Input: part model. Units: mm. Frame: model coordinates. Face numbers are marked on the shaded views. A direction names the side the tool comes from. Give positions to 0.01 mm unless a question says otherwise; leave off trailing zeros. Loops run counter-clockwise (first coordinate to the right, second up) from the corner with the lowest first, then second, coordinate; pieces in that order, holes last. Notation, with made-up numbers: (-30.5, 2.25) - (-2.5, 2.25) arc R13 ccw to (-2.5, 6.25) - close; hole circle Ø1 at (26.5, 12.25). An arc over 180 degrees is marked (long way). Answer as a JSON object with one key per item and string values. Group by question number.
(1) Mould query, pull axis X, two halves, no side actions, for the marked faces 4, 5, 6 and 7. Classes: +X half, -X half, draft (parallel to the pull), parting line (faces both ways), or undercut.
(2) Section query A-A (z = -12). Return loops of the section in (x, y).
(3) Access query for the marked faces 1, 2 and 3. Directions: +Z, -Z, +X, -X, +Y, -Y. A direction counts if a zero-diameter tool reaches every point of the face in a straight line with its end or side. Return the directions, or none.
(4) Pin query (flat end, axial travel): P1, Ø2, axis at x = 12.5, z = 15.5, coming from the -Y side; P2, Ø11.5, axis at y = 22.5, z = -2.5, coming from the -X side; P3, Ø12, axis at x = 37.5, z = -15, coming from the -Y side. Return the tip coordinate at first contact, or that it passes through.
(5) Section query B-B (y = 45.5). Return loops of the section in (x, z) (3 decimals), plus the area to 3 significant figures.
(6) Section query C-C (z = 0). Return loops of the section in (x, y) (3 decimals).
(7) Section query D-D (x = 5.5). Return loops of the section in (y, z).
(8) Material intervals for L1, parallel to Y at x = 45, z = 8; L2, parallel to X at y = 10, z = 6; L3, parallel to X at y = 19, z = -2, sorted ascending.
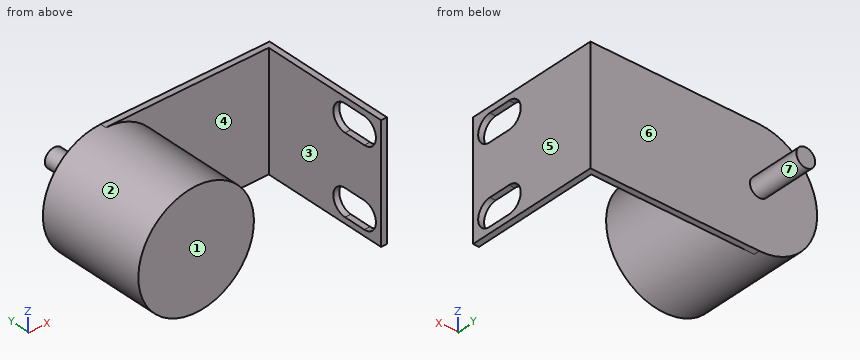
```python
from build123d import *

# Parameters (mm, degrees)
ESQUISSE1_R             = 19.5
BOSS_EXTRU_1_DEPTH      = 35
ESQUISSE2_R             = 3.175
BOSS_EXTRU_2_DEPTH      = 20
BOSS_EXTRU_3_DEPTH      = 2
ESQUISSE5_W             = 2
ESQUISSE5_H             = 39
BOSS_EXTRU_4_DEPTH      = 43.5
ENL_V_MAT_EXTRU_1_DEPTH = 5


with BuildPart() as part:
    # Esquisse1 → Boss.-Extru.1 (new body)
    with BuildSketch(Plane(origin=(0, 0, 0), x_dir=(1, 0, 0), z_dir=(0, 1, 0))):
        with Locations(Location((0, 0, 0), (0, 0, 270))):
            Circle(ESQUISSE1_R)
    extrude(amount=BOSS_EXTRU_1_DEPTH)

    # Esquisse2 → Boss.-Extru.2 (add)
    with BuildSketch(Plane(origin=(0, 35, 0), x_dir=(1, 0, 0), z_dir=(0, 1, 0))):
        with Locations(Location((0, 0, 0), (0, 0, 270))):
            Circle(ESQUISSE2_R)
    extrude(amount=BOSS_EXTRU_2_DEPTH)

    # Esquisse4 → Boss.-Extru.3 (add)
    with BuildSketch(Plane(origin=(0, 35, 0), x_dir=(1, 0, 0), z_dir=(0, 1, 0))):
        with BuildLine():
            Line((0, 19.5), (57, 19.5))
            Line((57, 19.5), (57, -19.5))
            Line((57, -19.5), (0, -19.5))
            ThreePointArc((0, -19.5), (-19.5, 0), (0, 19.5))
        make_face()
    extrude(amount=BOSS_EXTRU_3_DEPTH)

    # Esquisse5 → Boss.-Extru.4 (add)
    with BuildSketch(Plane.XZ.offset(-35)):
        with Locations((56, 0)):
            Rectangle(ESQUISSE5_W, ESQUISSE5_H)
    extrude(amount=BOSS_EXTRU_4_DEPTH)

    # Esquisse6 → Enlèv. mat.-Extru.1 (cut)
    with BuildSketch(Plane(origin=(57, 0, 0), x_dir=(0, 0, -1), z_dir=(1, 0, 0))):
        with BuildLine():
            Line((-8.5, 5.5), (-8.5, -2))
            ThreePointArc((-8.5, -2), (-13, -6.5), (-17.5, -2))
            Line((-17.5, -2), (-17.5, 5.5))
            ThreePointArc((-17.5, 5.5), (-13, 10), (-8.5, 5.5))
        make_face()
        with BuildLine():
            Line((8.5, 5.5), (8.5, -2))
            ThreePointArc((8.5, -2), (13, -6.5), (17.5, -2))
            Line((17.5, -2), (17.5, 5.5))
            ThreePointArc((17.5, 5.5), (13, 10), (8.5, 5.5))
        make_face()
    extrude(amount=-ENL_V_MAT_EXTRU_1_DEPTH, mode=Mode.SUBTRACT)


solid = part.part
```
Recorded:
{
 "1": {"face 4": "undercut", "face 5": "+X half", "face 6": "draft", "face 7": "parting line"},
 "2": {"outline": "(-15.37, 0) - (15.37, 0) - (15.37, 35) - (55, 35) - (55, 9.89) - (57, 9.89) - (57, 37) - (-15.37, 37) - close; (55, -8.5) - (57, -8.5) - (57, -6.39) - (55, -6.39) - close"},
 "3": {"face 1": "+Z, -Z, -X, -Y", "face 2": "-Y", "face 3": "+Z, -Z, -Y"},
 "4": {"P1": "stops at y = 0", "P2": "stops at x = -19.5", "P3": "stops at y = 35"},
 "5": {"outline": "circle Ø6.35 at (0, 0)", "area": "31.7 mm^2"},
 "6": {"outline": "(-19.5, 0) - (19.5, 0) - (19.5, 35) - (55, 35) - (55, -8.5) - (57, -8.5) - (57, 37) - (3.175, 37) - (3.175, 55) - (-3.175, 55) - (-3.175, 37) - (-19.5, 37) - close"},
 "7": {"outline": "(0, -18.71) - (35, -18.71) - (35, -19.5) - (37, -19.5) - (37, 19.5) - (35, 19.5) - (35, 18.71) - (0, 18.71) - close"},
 "8": {"L1": "y = 35 to 37", "L2": "x = -18.55 to 18.55, 55 to 57", "L3": "x = -19.4 to 19.4, 55 to 57"}
}
